For this review, take the finished solid that the model builds, in its own axes (mm). A direction names the side the tool comes from. Coordinates: 2 decimals unless noted, no trailing zeros. Write each loop counter-clockwise with the first axis right and the second up, starting at its lowest first coordinate (ties: lowest second). Pieces come first, ordered by that corner, then holes. Notation, with made-up numbers: (22, 37.5) -> (70, 37.5) arc R21 ccw to (70, 75.5) -> close; hole circle Ø3 at (57, 6). An arc over 180 degrees is marked (long way). One line per item, written item: value. Start each with the question number.
1) For probe 1 along Y at (x, z) = (0, 15) (3 decimals); probe 2 along Y at (x, z) = (0, 2.25) (3 decimals); probe 3 along Y at (x, z) = (-1.5, 2.5), list the stretches that pass through material, from the lowest coordinate up. Write a range as from..to.
2) Add section C-C (x = -8.25). State the section outline as (y, z) points, and give its area (3 significant figures).
3) For pin 1 Ø6 at (y, z) = (4, 12) entering from +X; pin 2 Ø5 at (y, z) = (6, 2.5) entering from +X; pin 3 Ø6 at (x, z) = (-1, 18) entering from +Y (3 decimals), all flat-tipped, find the tip position at first contact; note any pin that passes through.
4) Mouldability with a two-part tool opening along X and no side actions: class faces 3 (the flat face through (3, 7, -2.54)), 4 (the cylindrical face through (-1.377, 3.326, 11.306)), 5 (the cylindrical face through (1.73, 0.55, -0.04)) as released by +X, released by -X, zero draft, split by the parting line, or undercut.
5) Add section A-A (x = 0). State the section outline as (y, z) points (3 decimals), and give its area (3 significant figures).
6) Add section D-D (y = 3.75). State the section outline as (x, z) points, and give its area (3 significant figures).
7) Add section B-B (y = 10). State the section outline as (x, z) points, and give its area (3 significant figures).
8) Machinability: for faces 1 (the flat face through (-3, 14, 20.32)), 2 (the cylindrical face through (-1.71, 12.2, 9.98)), which of the approach directions +Z, -Z, +X, -X, +Y, -Y give a long, thin tool a straight path to every point of the face, cutting with its end or side? Answer none if there is none.
from build123d import *

# Parameters (mm, degrees)
SKETCH1_R           = 12.7
SKETCH1_R_2         = 1.8161
BOSS_EXTRUDE1_DEPTH = 2.54
SKETCH2_R           = 6.35
BOSS_EXTRUDE2_DEPTH = 20.32
SKETCH4_R           = 3.175
CUT_EXTRUDE1_DEPTH  = 37.061067996
CUT_EXTRUDE2_START  = -2.54
SKETCH5_R           = 6.35
SKETCH5_R_2         = 5.08
CUT_EXTRUDE2_DEPTH  = 2.54


with BuildPart() as part:
    # Sketch1 → Boss-Extrude1 (new, symmetric)
    with BuildSketch(Plane.XY):
        with Locations((0, 9.525)):
            Circle(SKETCH1_R)
        Circle(SKETCH1_R_2, mode=Mode.SUBTRACT)
        with Locations((-8.248891971, 14.2875)):
            Circle(SKETCH1_R_2, mode=Mode.SUBTRACT)
        with Locations((8.248891971, 14.2875)):
            Circle(SKETCH1_R_2, mode=Mode.SUBTRACT)
    extrude(amount=BOSS_EXTRUDE1_DEPTH, both=True)

    # Sketch2 → Boss-Extrude2 (add)
    with BuildSketch(Plane.XY.offset(2.54)):
        with Locations((0, 9.525)):
            Circle(SKETCH2_R)
    extrude(amount=BOSS_EXTRUDE2_DEPTH)

    # Sketch4 → Cut-Extrude1 (cut, through all)
    with BuildSketch(Plane(origin=(0, 0, -2.54), x_dir=(-1, 0, 0), z_dir=(0, 0, -1))):
        with Locations((0, 9.525)):
            Circle(SKETCH4_R)
    extrude(amount=-CUT_EXTRUDE1_DEPTH, mode=Mode.SUBTRACT)

    # Sketch5 → Cut-Extrude2 (cut)
    with BuildSketch(Plane.XY.offset(22.86).offset(CUT_EXTRUDE2_START)):
        with Locations((0, 9.525)):
            Circle(SKETCH5_R)
        with Locations((0, 9.525)):
            Circle(SKETCH5_R_2, mode=Mode.SUBTRACT)
    extrude(amount=CUT_EXTRUDE2_DEPTH, mode=Mode.SUBTRACT)


solid = part.part
Numbers:
1. probe 1: 3.175..6.35, 12.7..15.875
1. probe 2: -3.175..-1.816, 1.816..6.35, 12.7..22.225
1. probe 3: -3.09..-1.02, 1.02..6.73, 12.32..22.14
2. outline: (-0.13, -2.54) -> (12.47, -2.54) -> (12.47, 2.54) -> (-0.13, 2.54) -> close; (16.1, -2.54) -> (19.18, -2.54) -> (19.18, 2.54) -> (16.1, 2.54) -> close
2. area: 79.6 mm²
3. pin 1: x = 5.83
3. pin 2: x = 12.66
3. pin 3: y = 15.875
4. face 3: zero draft
4. face 4: split by the parting line
4. face 5: undercut
5. outline: (-3.175, -2.54) -> (-1.816, -2.54) -> (-1.816, 2.54) -> (-3.175, 2.54) -> close; (1.816, -2.54) -> (6.35, -2.54) -> (6.35, 22.86) -> (4.445, 22.86) -> (4.445, 20.32) -> (3.175, 20.32) -> (3.175, 2.54) -> (1.816, 2.54) -> close; (12.7, -2.54) -> (22.225, -2.54) -> (22.225, 2.54) -> (15.875, 2.54) -> (15.875, 20.32) -> (14.605, 20.32) -> (14.605, 22.86) -> (12.7, 22.86) -> close
5. area: 201 mm²
6. outline: (-11.31, -2.54) -> (11.31, -2.54) -> (11.31, 2.54) -> (2.64, 2.54) -> (2.64, 20.32) -> (-2.64, 20.32) -> (-2.64, 2.54) -> (-11.31, 2.54) -> close
6. area: 209 mm²
7. outline: (-12.69, -2.54) -> (-3.14, -2.54) -> (-3.14, 22.86) -> (-5.06, 22.86) -> (-5.06, 20.32) -> (-6.33, 20.32) -> (-6.33, 2.54) -> (-12.69, 2.54) -> close; (3.14, -2.54) -> (12.69, -2.54) -> (12.69, 2.54) -> (6.33, 2.54) -> (6.33, 20.32) -> (5.06, 20.32) -> (5.06, 22.86) -> (3.14, 22.86) -> close
7. area: 220 mm²
8. face 1: +Z
8. face 2: +Z, -Z
